```python
from build123d import *

# Parameters (mm, degrees)
SKICA2_R                = 4
P_IDAT_VYSUNUT_M1_DEPTH = 7


with BuildPart() as part:
    # Skica2 → Přidat vysunutím1 (new body)
    with BuildSketch(Plane.XY):
        with BuildLine():
            Line((-52.88, 7.463618425), (-9.36, 24.256759883))
            ThreePointArc((-9.36, 24.256759883), (25.371520283, 5.682073435), (1.88, -25.931941694))
            ThreePointArc((1.88, -25.931941694), (6.44926926, -13.322161987), (8, 0))
            ThreePointArc((8, 0), (0, 8), (-8, 0))
            ThreePointArc((-8, 0), (-9.635178846, -11.60522353), (-14.413391103, -22.306798678))
            Line((-14.413391103, -22.306798678), (-52.88, -7.463618425))
            ThreePointArc((-52.88, -7.463618425), (-58, 0), (-52.88, 7.463618425))
        make_face()
        with Locations((-50, 0)):
            Circle(SKICA2_R, mode=Mode.SUBTRACT)
    extrude(amount=P_IDAT_VYSUNUT_M1_DEPTH)


solid = part.part
```
Can you work these out from the model? Positions are in its coordinate system, mm. A direction names the side the tool comes from. Give positions to 0.01 mm unless a question says otherwise; leave off trailing zeros. Order: outer loops, then holes, each group sorted by start corner. A loop starts at its lowest first (then second) coordinate and runs counter-clockwise, first axis right, second up. Notation, with made-up numbers: (-4, 2) - (11, 2) arc R19 ccw to (11, 23) - close; hole circle Ø10 at (73, 37). An arc over 180 degrees is marked (long way). Use a Markdown table: item, result. Add a question column.
Q1. If we section it at C-C on x = -52: Write out the boundary of the cut face in (y, z).
Q2. If we mould it in two halves opening along Y, with no side actions, what happens to faces 3 (the flat face through (-31.425, 15.743, 3.451)), 4 (the cylindrical face through (-9.59, -11.45, 3.45)), 5 (the cylindrical face through (6.406, -13.505, 3.451))? For each: released by +Y, released by -Y, zero draft, split by the parting line, or undercut.
Q3. Please list where these lines run through material, in increasing order: line 1 along X through (y, z) = (-3, 5.25); line 2 along X through (y, z) = (-1, 2.5); line 3 along Y through (x, z) = (-0.5, 2.25).
Q4. If we section it at A-A on z = 5: Write out the boundary of the cut face in (x, y).
Q5. If we section it at B-B on y = -19: Write out the boundary of the cut face in (x, z).
Q6. If we section it at D-D on y = 2: Write out the boundary of the cut face in (x, z), plus the area to 3 significant figures.
Q7. On a 3-axis mill with a long thin cutter (end or side, diameter ignored), from which of +Z, -Z, +X, -X, +Y, -Y can I reach the whole of each face in a straight line? I mean faces 1 (the cylindrical face through (0, 8, 3)), 2 (the flat face through (-33.38, -14.99, 3.45)). Say none if no direction works.
Q8. I'm going to push flat-ended pins straight in: pin 1 (1.5 mm diameter, centred on x = 13, z = 5.5, fed in from +Y); pin 2 (4 mm diameter, centred on x = -7.5, z = 6, fed in from +Y); pin 3 (1.5 mm diameter, centred on y = 4, z = 5, fed in from +X); pin 4 (7 mm diameter, centred on x = -50, y = 0, fed in from -Z). Where does each tip first touch, or does it pass through?
Answers follow:
| question | item | result |
|---|---|---|
| 1 | outline | (-7.8, 0) - (-3.46, 0) - (-3.46, 7) - (-7.8, 7) - close; (3.46, 0) - (7.8, 0) - (7.8, 7) - (3.46, 7) - close |
| 2 | face 3 | released by +Y |
| 2 | face 4 | released by -Y |
| 2 | face 5 | undercut |
| 3 | line 1 | x = -57.42 to -52.65, -47.35 to -8.11, 7.92 to 25.83 |
| 3 | line 2 | x = -57.94 to -53.87, -46.13 to -8.01, 7.99 to 25.98 |
| 3 | line 3 | y = 7.98 to 26 |
| 4 | outline | (-52.88, -7.46) - (-14.41, -22.31) arc R42 ccw to (-8, 0) arc R8 cw to (8, 0) arc R58 cw to (1.88, -25.93) arc R26 ccw (long way) to (-9.36, 24.26) - (-52.88, 7.46) arc R8 ccw to start; hole circle Ø8 at (-50, 0) |
| 5 | outline | (-22.98, 0) - (-12.54, 0) - (-12.54, 7) - (-22.98, 7) - close; (4.8, 0) - (17.75, 0) - (17.75, 7) - (4.8, 7) - close |
| 6 | outline | (-57.75, 0) - (-53.46, 0) - (-53.46, 7) - (-57.75, 7) - close; (-46.54, 0) - (-7.75, 0) - (-7.75, 7) - (-46.54, 7) - close; (7.75, 0) - (25.92, 0) - (25.92, 7) - (7.75, 7) - close |
| 6 | area | 429 mm^2 |
| 7 | face 1 | +Z, -Z |
| 7 | face 2 | +Z, -Z, -X, -Y |
| 8 | pin 1 | stops at y = 22.93 |
| 8 | pin 2 | stops at y = 25.41 |
| 8 | pin 3 | stops at x = 25.8 |
| 8 | pin 4 | passes through |
